Read the model definition and answer for the solid it produces. Units are mm, in the model's axes. Give positions to 0.01 mm unless a question says otherwise; leave off trailing zeros. Order: outer loops, then holes, each group sorted by start corner. A loop starts at its lowest first (then second) coordinate and runs counter-clockwise, first axis right, second up.
Item 1: A cutting plane is placed at C-C (z = 3.3). State how many separate pieces and enclosed holes the cut face has, plus the area to 3 significant figures.
Item 2: A cutting plane is placed at A-A (y = 180). Write down the section's boundary in (x, z), plus the area to 3 significant figures.
Item 3: Find the intervals of material crossed by line 1 along Y through (x, z) = (180, 1.4); line 2 along Y through (x, z) = (181.5, 1.6); line 3 along X through (y, z) = (182, 2.4), in increasing order.
Item 4: A cutting plane is placed at D-D (y = 44). Write down the section's boundary in (x, z), plus the area to 3 significant figures.
Item 5: A cutting plane is placed at B-B (x = 180). Write down the section's boundary in (y, z).
Item 6: Given pin 1 Ø1 at (x, z) = (67, 1.5) entering from -Y; pin 2 Ø1 at (y, z) = (46, 3.5) entering from -X; pin 3 Ø1.2 at (x, z) = (60, 1.5) entering from +Y, each flat-ended and moving along its own axis, determine where each tip first touches the part or whether it passes through.
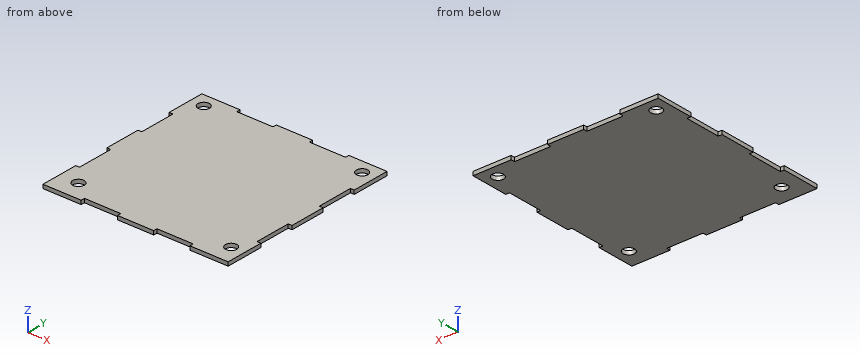
from build123d import *

# Parameters (mm, degrees)
F1_DEPTH = 4
F2_R     = 6
F3_DEPTH = 4


with BuildPart() as f1:
    # F0 (on Top) → F1 (new body)
    with BuildSketch(Plane.XY):
        Polygon((0, 40), (0, 0), (40, 0), (40, 4), (78, 4), (78, 0), (116, 0), (116, 4), (154, 4), (154, 0), (194, 0), (194, 40), (190, 40), (190, 78), (194, 78), (194, 116), (190, 116), (190, 154), (194, 154), (194, 194), (154, 194), (154, 190), (116, 190), (116, 194), (78, 194), (78, 190), (40, 190), (40, 194), (0, 194), (0, 154), (4, 154), (4, 116), (0, 116), (0, 78), (4, 78), (4, 40), align=None)
    extrude(amount=F1_DEPTH)

    # F2 (on face) → F3 (cut)
    with BuildSketch(Plane.XY.offset(4)):
        with Locations((14, 180)):
            Circle(F2_R)
        with Locations((180, 180)):
            Circle(F2_R)
        with Locations((180, 20)):
            Circle(F2_R)
        with Locations((20, 20)):
            Circle(F2_R)
    extrude(amount=-F3_DEPTH, mode=Mode.SUBTRACT)


solid = f1.part
Response values:
1. separate pieces: 1
1. enclosed holes: 4
1. area: 36,000 mm2
2. outline: (0, 0) - (8, 0) - (8, 4) - (0, 4) - close; (20, 0) - (174, 0) - (174, 4) - (20, 4) - close; (186, 0) - (194, 0) - (194, 4) - (186, 4) - close
2. area: 680 mm2
3. line 1: y = 0 to 14, 26 to 174, 186 to 194
3. line 2: y = 0 to 14.19, 25.81 to 174.19, 185.81 to 194
3. line 3: x = 0 to 8.34, 19.66 to 174.34, 185.66 to 194
4. outline: (4, 0) - (190, 0) - (190, 4) - (4, 4) - close
4. area: 744 mm2
5. outline: (0, 0) - (14, 0) - (14, 4) - (0, 4) - close; (26, 0) - (174, 0) - (174, 4) - (26, 4) - close; (186, 0) - (194, 0) - (194, 4) - (186, 4) - close
6. pin 1: stops at y = 4
6. pin 2: stops at x = 4
6. pin 3: stops at y = 190
